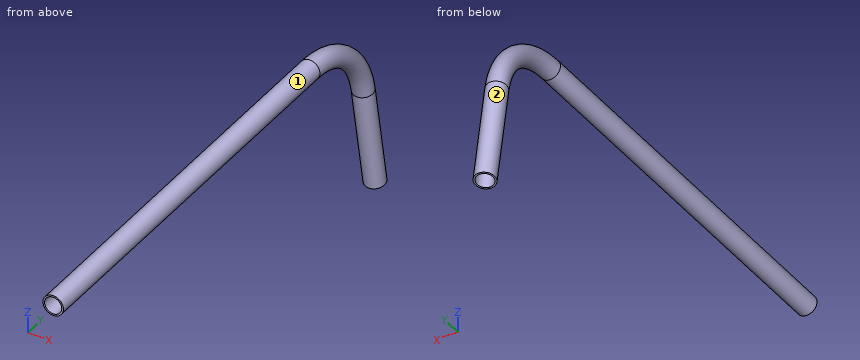
```python
from build123d import *

# Parameters (mm, degrees)
SKETCH1_R           = 3.175
SKETCH1_R_2         = 2.667
BOSS_EXTRUDE1_DEPTH = 127
SKETCH3_R           = 3.175
SKETCH3_R_2         = 2.667


with BuildPart() as part:
    # Sketch1 → Boss-Extrude1 (new body)
    with BuildSketch(Plane(origin=(0, 0, 0), x_dir=(1, 0, 0), z_dir=(0, 1, 0))):
        Circle(SKETCH1_R)
        Circle(SKETCH1_R_2, mode=Mode.SUBTRACT)
    extrude(amount=BOSS_EXTRUDE1_DEPTH)

    # Sweep1: sweep along a path in Sketch2
    with BuildLine(Plane(origin=(0, 0, 0), x_dir=(0, 0, -1), z_dir=(1, 0, 0))) as sweep1_path:
        Line((55.012797254, 159.298316562), (22.166564651, 153.456678788))
        ThreePointArc((22.166564651, 153.456678788), (6.2740832, 144.25769713), (0, 127))
    # Sketch3 → Sweep1 (sweep)
    with BuildSketch(Plane(origin=(0, 127, 0), x_dir=(1, 0, 0), z_dir=(0, 1, 0))):
        Circle(SKETCH3_R)
        Circle(SKETCH3_R_2, mode=Mode.SUBTRACT)
    sweep(path=sweep1_path.line)


solid = part.part
```
Here's how the part is built. I have some questions about the finished solid (model axes, mm). Face numbers are marked on the shaded views. A direction names the side the tool comes from. Round coordinates to 2 decimals unless told otherwise and drop trailing zeros. Loops run counter-clockwise (first coordinate to the right, second up) from the corner with the lowest first, then second, coordinate; pieces in that order, holes last. Notation, with made-up numbers: (33.25, 51.25) -> (59.25, 51.25) arc R13 cw to (59.25, 56.25) -> close; hole circle Ø4 at (89.5, -27). An arc over 180 degrees is marked (long way). Answer as CSV lines item,"result". Start each with the question number.
1. Imagine slicing it at B-B on y = 81. Write out the boundary of the cut face in (x, z) (3 decimals), plus the area to 3 significant figures.
2. I'm going to push flat-ended pins straight in: P1, Ø1.5, axis at x = 1, y = 95.5, coming from the -Z side; P2, Ø1.5, axis at x = -0.5, z = -18, coming from the +Y side; P3, Ø10, axis at y = 115, z = -5, coming from the +X side (3 decimals). Where does each tip first touch, or does it pass through?
3. For the marked faces 1 and 2, which set-ups out of +Z, -Z, +X, -X, +Y, -Y let a thin tool reach every point of the face, with its end or its side?
4. I need wall thicknesses on probe 1 along Z at (x, y) = (0, 34) (3 decimals); probe 2 along Y at (x, z) = (0.5, -24.5). Which ranges of each line are inside material? Lowest first, please. Write a range as from..to.
5. Imagine slicing it at A-A on x = 0. Write out the boundary of the cut face in (y, z) (1 decimal), plus the area to 3 significant figures.
Solution:
1,outline,"circle Ø6.35 at (0, 0); hole circle Ø5.334 at (0, 0)"
1,area,"9.32 mm²"
2,P1,"z = -3.17"
2,P2,"y = 155.91"
2,P3,"x = 3.175"
3,face 1,"-Y"
3,face 2,"none"
4,probe 1,"-3.175..-2.667, 2.667..3.175"
4,probe 2,"150.69..151.21, 156.53..157.06"
5,outline,"(0, -3.2) -> (127, -3.2) arc R23.7 cw to (150.3, -22.7) -> (156.2, -55.6) -> (156.7, -55.5) -> (150.8, -22.6) arc R24.2 ccw to (127, -2.7) -> (0, -2.7) -> close; (0, 2.7) -> (127, 2.7) arc R29.5 cw to (156.1, -21.7) -> (161.9, -54.5) -> (162.4, -54.5) -> (156.6, -21.6) arc R30 ccw to (127, 3.2) -> (0, 3.2) -> close"
5,area,"201 mm²"
